Source: CAD feature listing. Evaluate the final solid. Frame: model axes, mm. Give positions to 0.01 mm unless a question says otherwise; leave off trailing zeros. Loops run counter-clockwise (first coordinate to the right, second up) from the corner with the lowest first, then second, coordinate; pieces in that order, holes last.
Autodesk Fusion 360 part; units mm, degrees
sketch "Esboço1" plane through (0, 0, 0) normal (0, 0, 1) x (1, 0, 0)
  line L0 (0, -37.25) -> (5.7315, -37.25)
  line L1 (0, -37.25) -> (-28.8244, -37.25)
  line L2 (13.7313, -37.25) -> (13.7313, -38.25)
  line L3 (13.7313, -38.25) -> (6.7313, -38.25)
  line L4 (6.7313, -38.25) -> (5.7315, -37.2502)
  line L5 (-33.6257, -26.0014) -> (-36.7371, -27.7066)
  line L6 (-27.7171, -34.088) -> (-28.9918, -35.3012)
  arc A0 (-31.1987, -35.48) -> (-30.9824, -35.4754) centre (-31.1987, -30.43) ccw
  arc A1 (-27.7171, -34.088) -> (-33.6257, -26.0014) centre (-31.1987, -30.43) ccw
  arc A2 (-31.1987, -35.2853) -> (-30.9824, -35.4754) centre (0, 0) ccw
  arc A3 (-28.8969, -37.1938) -> (-28.8244, -37.25) centre (0, 0) ccw
  arc A4 (-28.9918, -35.3012) -> (-28.8969, -37.1938) centre (-28.13, -36.2067) ccw
  arc A5 (-38.3557, -27.3358) -> (-36.7371, -27.7066) centre (-37.3378, -26.6104) ccw
  line L7 (13.7313, -45.25) -> (13.7313, -37.25)
  line L8 (13.7313, -30.43) -> (13.7313, 24.9988)
  line L9 (5.7315, -37.2502) -> (5.7315, -37.25)
  line L10 (13.7313, -37.25) -> (13.7313, -30.43)
  line L11 (6.7313, -38.25) -> (6.7313, -45.25)
  line L12 (6.7313, -45.25) -> (13.7313, -45.25)
  arc A6 (-34.0426, 26.2669) -> (-27.4054, 33.7737) centre (-31.1987, 30.44) ccw
  line L13 (-28.9198, 35.4969) -> (-27.4054, 33.7737)
  line L14 (-36.4461, 27.9049) -> (-34.0426, 26.2669)
  arc A7 (4.963, 46.8378) -> (-28.7437, 37.3123) centre (0, 0) ccw
  arc A8 (-38.1628, 27.6045) -> (-38.3557, -27.3358) centre (0, 0) ccw
  arc A9 (-28.7437, 37.3123) -> (-28.9198, 35.4969) centre (-27.9809, 36.3221) ccw
  arc A10 (-36.4461, 27.9049) -> (-38.1628, 27.6045) centre (-37.15, 26.8719) ccw
  line L15 (13.7313, 24.9988) -> (12.7371, 25.9986)
  line L16 (12.7371, 25.9986) -> (6.8571, 25.9986)
  line L17 (6.8571, 25.9986) -> (5.8601, 26.9956)
  line L18 (5.8601, 26.9956) -> (5.8601, 45.6356)
  line L19 (5.8601, 45.6356) -> (4.963, 46.8378)
  line L20 (5.8601, 40.1056) -> (-1.1399, 40.1056)
  line L21 (-1.1399, 40.1056) -> (-1.1399, 47.0862)
  line L22 (-46.9419, 3.8556) -> (-39.9419, 3.8556)
  line L23 (-39.9419, 3.8556) -> (-39.9419, -3.1444)
  line L24 (-39.9419, -3.1444) -> (-46.9949, -3.1444)
  circle A11 centre (-43.4419, 0) radius 2
  circle A12 centre (-43.4419, 0) radius 1.125
  circle A13 centre (10.2313, -41.75) radius 2
  circle A14 centre (10.2313, -41.75) radius 1.125
  circle A15 centre (2.3601, 43.6056) radius 2
  circle A16 centre (2.3601, 43.6056) radius 1.125
  dimension "d1" = 94.2
  dimension "d3" = 37.25
  dimension "d5" = 1
  dimension "d6" = 7
  dimension "d7" = 1.414
  dimension "d8" = 135
  dimension "d9" = 44.93
  dimension "d11" = 10.1
  dimension "d12" = 1.25
  dimension "d13" = 1.25
  dimension "d14" = 7
  dimension "d16" = 60.87
  dimension "d17" = 10.1
  dimension "d18" = 1.25
  dimension "d19" = 1.25
  dimension "d21" = 1.41
  dimension "d22" = 5.88
  dimension "d23" = 1.41
  dimension "d24" = 135
  dimension "d25" = 18.64
  dimension "d26" = 1.5
  dimension "d28" = 7
  dimension "d30" = 7
  dimension "d31" = 7
  dimension "d32" = 7.053
  dimension "d34" = 4
  dimension "d35" = 2.25
  dimension "d38" = 4
  dimension "d39" = 2.25
  dimension "d41" = 4
  dimension "d42" = 2.25
extrude "Extrusão1" add sketch "Esboço1" along normal blind 1 contours L0 L1 L2 L3 L4 L5 L6 A1 A3 A4 A5 L7 L8 L10 A6 L13 L14 A7 A8 A9 A10 L15 L16 L17 L18 L20 L21 L22 L23 L24
extrude "Extrusão2" add sketch "Esboço1" along normal blind 3.75 contours A8 L22 L23 L24 | A11
extrude "Extrusão3" cut sketch "Esboço1" along normal blind 3 contours A11
extrude "Extrusão4" add sketch "Esboço1" along normal blind 3.75 contours L3 L7 L11 L12 | A13
extrude "Extrusão5" cut sketch "Esboço1" along normal blind 3 contours A13
extrude "Extrusão6" add sketch "Esboço1" along normal blind 3.75 contours A7 L18 L19 L20 L21 | A15
extrude "Extrusão7" cut sketch "Esboço1" along normal blind 3 contours A15
chamfer "Chanfro1" distance 1 angle 45 1 edges at (13.7313, -45.25, 1.875)
chamfer "Chanfro2" distance 1 angle 45 1 edges at (6.7313, -45.25, 1.875)
equation "d1 = ( 47.1 * 2 ) * 1 mm"
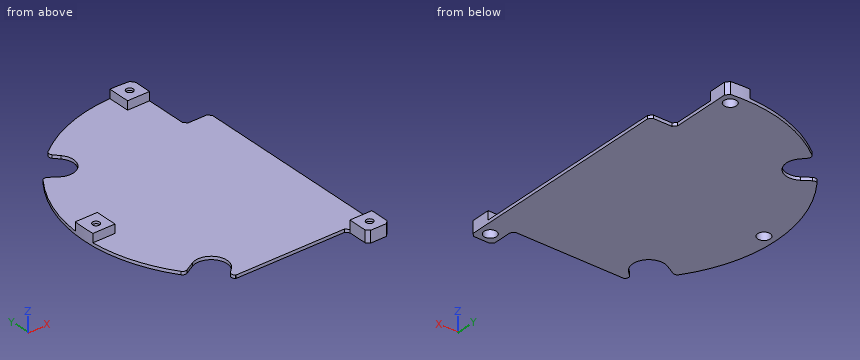
(1) Ray query, line 1 along Z through (x, y) = (-39, 19); line 2 along Y through (x, z) = (0, 1.7); line 3 along Y through (x, z) = (8, 2.05). Return the intervals inside material, ascending.
A:
line 1: z = 0 to 1
line 2: y = 40.11 to 47.1
line 3: y = -45.25 to -38.25
(2) Section C-C, the plane y = -41.75. Return the cut outline in (x, z).
A:
outline: (6.73, 0) - (8.23, 0) - (8.23, 3) - (9.11, 3) - (9.11, 3.75) - (6.73, 3.75) - close; (11.36, 3) - (12.23, 3) - (12.23, 0) - (13.73, 0) - (13.73, 3.75) - (11.36, 3.75) - close
(3) First-contact query: pin 1 (2 mm diameter, centred on y = 36.5, z = 3, fed in from +X); pin 2 (1.4 mm diameter, centred on x = 2, z = 2, fed in from -Y); pin 3 (0.5 mm diameter, centred on x = 9.5, z = 0.5, fed in from +Y); pin 4 (2.5 mm diameter, centred on x = 2.36, y = 43.61, fed in from -Z). Flat tips, straight axial feed; report the tip coordinate or a pass-through.
A:
pin 1: passes through
pin 2: stops at y = 40.11
pin 3: stops at y = 26
pin 4: stops at z = 3
(4) Section D-D, the plane x = -16.5. Return the cut outline in (y, z).
A:
outline: (-37.25, 0) - (44.12, 0) - (44.12, 1) - (-37.25, 1) - close
(5) Section A-A, the plane y = 0. Return the cut outline in (x, z).
A:
outline: (-47.1, 0) - (-45.44, 0) - (-45.44, 3) - (-44.57, 3) - (-44.57, 3.75) - (-47.1, 3.75) - close; (-42.32, 3) - (-41.44, 3) - (-41.44, 0) - (13.73, 0) - (13.73, 1) - (-39.94, 1) - (-39.94, 3.75) - (-42.32, 3.75) - close
(6) Section B-B, the plane z = 2. Return the cut outline in (x, y), then the cut area to 3 significant figures.
A:
outline: (-46.99, -3.14) - (-39.94, -3.14) - (-39.94, 3.86) - (-46.94, 3.86) arc R47.1 ccw to start; (-1.14, 40.11) - (5.86, 40.11) - (5.86, 45.64) - (4.96, 46.84) arc R47.1 ccw to (-1.14, 47.09) - close; (6.73, -44.25) - (7.73, -45.25) - (12.73, -45.25) - (13.73, -44.25) - (13.73, -38.25) - (6.73, -38.25) - close; hole circle Ø4 at (-43.44, 0); hole circle Ø4 at (2.36, 43.61); hole circle Ø4 at (10.23, -41.75)
area: 108 mm2
